The listing builds one solid part. Answer for the finished solid, in the listing's coordinates (mm). A direction names the side the tool comes from. Coordinates: 2 decimals unless noted, no trailing zeros. Write each loop counter-clockwise with the first axis right and the second up, starting at its lowest first coordinate (ties: lowest second). Pieces come first, ordered by that corner, then holes.
(1) For a pull along Y with two mould halves and no side action, classify faces 1 (the flat face through (370, 20, 0)), 2 (the flat face through (751, -2, -19)), 3 (the flat face through (370, 0, 18)) as +Y half, -Y half, draft (parallel to the pull), parting line (faces both ways), or undercut.
(2) The part is cut by section A-A on y = 1. Determine the outline of the cut face in (x, z), plus the area to 3 significant figures.
(3) The part is cut by section C-C on x = 294. Determine the outline of the cut face in (y, z).
(4) Which of the six approach directions +Z, -Z, +X, -X, +Y, -Y give full straight-line access (tool end or side, diameter ignored) to faces 4 (the flat face through (370, 18, 0)), 5 (the flat face through (370, 0, -20))?
(5) Straight lines are drawn through the part: line 1 (Z direction, x = 279, y = 15); line 2 (Z direction, x = 2, y = -19). For each, find the intervals that lie inside material, in ascending order.
from build123d import *

# Parameters (mm, degrees)
F0_W     = 40
F0_H     = 40
F0_W_2   = 36
F0_H_2   = 36
F1_DEPTH = 751
F3_D     = 3
F3_DEPTH = 50


with BuildPart() as f1:
    # F0 (on Right) → F1 (new body)
    with BuildSketch(Plane.YZ):
        Rectangle(F0_W, F0_H)
        Rectangle(F0_W_2, F0_H_2, mode=Mode.SUBTRACT)
    extrude(amount=F1_DEPTH)

    # F3
    with Locations(Plane(origin=(0, 20, 0), x_dir=(-1, 0, 0), z_dir=(0, 1, 0))):
        with Locations((-748.5, -7.73), (-738.5, -7.73), (-2.5, -7.73), (-12.5, -7.73)):
            Hole(F3_D / 2, depth=F3_DEPTH)


solid = f1.part
Model answer:
1. face 1: +Y half
1. face 2: draft
1. face 3: undercut
2. outline: (0, -20) - (751, -20) - (751, -18) - (0, -18) - close; (0, 18) - (751, 18) - (751, 20) - (0, 20) - close
2. area: 3,000 mm2
3. outline: (-20, -20) - (20, -20) - (20, 20) - (-20, 20) - close; hole (-18, -18) - (18, -18) - (18, 18) - (-18, 18) - close
4. face 4: +X, -X
4. face 5: -Z, +X, -X, +Y, -Y
5. line 1: z = -20 to -18, 18 to 20
5. line 2: z = -20 to -9.14, -6.32 to 20
